```python
from build123d import *

# Parameters (mm, degrees)
F1_DEPTH = 127
F2_R     = 44.45
F3_R     = 23.0505
F3_R_2   = 19.3675
F4_DEPTH = 76.2


with BuildPart() as f1:
    # F0 (on Front) → F1 (new body, symmetric)
    with BuildSketch(Plane.XZ):
        Polygon((-127, -127), (0, -127), (127, -127), (127, 254), (-127, 254), align=None)
    extrude(amount=F1_DEPTH, both=True)

    # F2
    f2_edges = [f1.edges().sort_by_distance(p)[0] for p in [
        (0, -127, 254),
        (127, 0, 254),
        (0, -127, -127),
        (127, -127, 63.5),
        (-127, -127, 63.5),
        (127, 0, -127),
        (0, 127, 254),
        (-127, 0, 254),
        (-127, 127, 63.5),
        (-127, 0, -127),
        (0, 127, -127),
        (127, 127, 63.5),
    ]]
    fillet(f2_edges, radius=F2_R)

    # F3 (on face) → F4 (join)
    with BuildSketch(Plane.XZ.offset(127)):
        with Locations((0, -41.275)):
            Circle(F3_R)
        with Locations((0, -41.275)):
            Circle(F3_R_2, mode=Mode.SUBTRACT)
    extrude(amount=F4_DEPTH)


solid = f1.part
```
Verification items for the finished model (mm, model axes). A direction names the side the tool comes from. Round coordinates to 2 decimals unless told otherwise and drop trailing zeros. Write each loop counter-clockwise with the first axis right and the second up, starting at its lowest first coordinate (ties: lowest second). Pieces come first, ordered by that corner, then holes.
1. Section check B-B on x = 76. Enter the section's corners in (y, z).
2. Gauge pin test, flat ends, axial feed: P1, Ø11.5, axis at x = 3, z = -42, coming from the -Y side; P2, Ø1, axis at x = 71.5, y = -122, coming from the -Z side; P3, Ø1.5, axis at y = -83.5, z = 85.5, coming from the +X side. Record the tip position at first contact, or that the pin passes through.
3. Scan lines: L1, parallel to Z at x = 0, y = -160; L2, parallel to Y at x = 51, z = -60; L3, parallel to X at y = -76.5, z = -85. Record each from-to range of solid material in increasing order.
4. Access from +Z, -Z, +X, -X, +Y, -Y to the whole of each face (thin tool, end or side, straight path). Record for faces 1 (the flat face through (-5, -203.2, -22)), 2 (the cylindrical face through (10.636, -164.567, -61.725)).
5. Draft check along X on faces 3 (the cylindrical face through (-1.156, -113.633, 241.325)), 4 (the cylindrical face through (113.633, -1.156, 241.325)), 5 (the cylindrical face through (-114.325, 1.156, 240.633)), 6 (the cylindrical face through (-15.37, -164.57, -53.06)). Enter one of: +X half, -X half, draft (parallel to the pull), parting line (faces both ways), or undercut.
6. Section check C-C on x = 0. Enter the section's corners in (y, z), plus the area to 3 significant figures.
7. Section check D-D on y = -147.5. Enter the section's corners in (x, z) (1 decimal), plus the area to 3 significant figures.
8. Section check A-A on z = 178.5. Enter the section's corners in (x, y).
Answer:
1. outline: (-127, -82.55) arc R44.45 ccw to (-82.55, -127) - (82.55, -127) arc R44.45 ccw to (127, -82.55) - (127, 209.55) arc R44.45 ccw to (82.55, 254) - (-82.55, 254) arc R44.45 ccw to (-127, 209.55) - close
2. P1: stops at y = -127
2. P2: stops at z = -103.97
2. P3: stops at x = 127
3. L1: z = -64.33 to -60.64, -21.91 to -18.22
3. L2: y = -127 to 127
3. L3: x = -126.93 to 126.93
4. face 1: +Z, -Z, +X, -X, -Y
4. face 2: -Y
5. face 3: draft
5. face 4: +X half
5. face 5: -X half
5. face 6: undercut
6. outline: (-203.2, -64.33) - (-127, -64.33) - (-127, -82.55) arc R44.45 ccw to (-82.55, -127) - (82.55, -127) arc R44.45 ccw to (127, -82.55) - (127, 209.55) arc R44.45 ccw to (82.55, 254) - (-82.55, 254) arc R44.45 ccw to (-127, 209.55) - (-127, -18.22) - (-203.2, -18.22) - (-203.2, -21.91) - (-127, -21.91) - (-127, -60.64) - (-203.2, -60.64) - close
6. area: 95,600 mm2
7. outline: circle Ø46.1 at (0, -41.3); hole circle Ø38.7 at (0, -41.3)
7. area: 491 mm2
8. outline: (-127, -82.55) arc R44.45 ccw to (-82.55, -127) - (82.55, -127) arc R44.45 ccw to (127, -82.55) - (127, 82.55) arc R44.45 ccw to (82.55, 127) - (-82.55, 127) arc R44.45 ccw to (-127, 82.55) - close
